Geometry: final body of the model. Coordinates: model frame, mm. A direction names the side the tool comes from. Give positions to 0.01 mm unless a question says otherwise; leave off trailing zeros. Write each loop counter-clockwise with the first axis right and the second up, starting at its lowest first coordinate (ties: lowest second). Pieces come first, ordered by that corner, then holes. Notation, with made-up numbers: M 4.25,62.5 L 52.25,62.5 A21 ccw 52.25,94.5 Z; hole C 22.25,-9 d9. An arc over 180 degrees is marked long. Use a Markdown table: item, result. Add a question column.
(1) Reachability of faces 4 (the cylindrical face through (37.79, -108.4, -99.58)), 5 (the flat face through (60.5, 27, 41)), 6 (the flat face through (11, -2, 150)), 7 (the cylindrical face through (36.1, -77.8, -98.3)), 8 (the cylindrical face through (20.706, -27.169, 86.273)) from +Z, -Z, +X, -X, +Y, -Y: full face, straight path, thin tool, end or side. Return the list, or none.
(2) Pin query (flat end, axial travel): pin 1 Ø3 at (x, y) = (49, -29.5) entering from -Z; pin 2 Ø2 at (x, y) = (24.5, 78) entering from +Z; pin 3 Ø3.5 at (x, z) = (40, 120) entering from +Y. Return the tip coordinate at first contact, or that it passes through.
(3) Cut plane B-B (x = 30). Output: boundary loops of the cut face in (y, z).
(4) Cut plane C-C (z = 32.5). Output: boundary loops of the cut face in (x, y), plus the area to 3 significant figures.
(5) Material intervals for L1, parallel to Z at x = 40, y = -106; L2, parallel to Y at x = 4, z = 0 (3 decimals); L3, parallel to X at y = -108, z = -97, sorted ascending.
(6) Cut plane A-A (y = 0). Output: boundary loops of the cut face in (x, z), plus the area to 3 significant figures.
(7) Cut plane D-D (y = -57.5). Output: boundary loops of the cut face in (x, z).
(8) Draft query along Z for faces 1 (the conical face through (38.568, -75.483, -82.06)), 2 (the conical face through (16.49, 69.66, -82.98)), 3 (the cylindrical face through (37.85, 98.07, -98.34)). Return one class per face: released by +Z, released by -Z, zero draft, split by the parting line, or undercut.
```python
from build123d import *

# Parameters (mm, degrees)
SKETCH1_W                 = 300
SKETCH1_H                 = 260
BOSS_EXTRUDE1_DEPTH       = 60.5
SKETCH2_R                 = 90.45
CUT_EXTRUDE1_DEPTH        = 42
SKETCH9_R                 = 41.51
CUT_EXTRUDE9_DEPTH        = 306
SKETCH12_W                = 39
SKETCH12_H                = 260
CUT_EXTRUDE12_DEPTH       = 14
SKETCH13_W                = 39
SKETCH13_H                = 260
CUT_EXTRUDE13_DEPTH       = 36.45
SKETCH14_W                = 39
SKETCH14_H                = 14
CUT_EXTRUDE14_DEPTH       = 333.506014983
SKETCH15_W                = 22.45
SKETCH15_H                = 260
CUT_EXTRUDE15_DEPTH       = 208.50963833
F_6_0MM_DOWEL_HOLE1_D     = 6
F_6_0MM_DOWEL_HOLE1_DEPTH = 30
F_6_0MM_DOWEL_HOLE1_TIP   = 1.802581857
F_6_0MM_DOWEL_HOLE2_D     = 6
F_6_0MM_DOWEL_HOLE2_DEPTH = 30
F_6_0MM_DOWEL_HOLE2_TIP   = 1.802581857
F_6_0MM_DOWEL_HOLE3_D     = 6
F_6_0MM_DOWEL_HOLE3_DEPTH = 15
F_6_0MM_DOWEL_HOLE3_TIP   = 1.802581857
SKETCH25_W                = 39
SKETCH25_H                = 14
CUT_EXTRUDE16_DEPTH       = 333.506014983
SKETCH26_W                = 257.55
SKETCH26_H                = 240
CUT_EXTRUDE18_DEPTH       = 2.3
F_6_0MM_DOWEL_HOLE4_D     = 6
F_6_0MM_DOWEL_HOLE4_DEPTH = 15
F_6_0MM_DOWEL_HOLE4_TIP   = 1.802581857
SKETCH32_R                = 2.25
CUT_EXTRUDE19_DEPTH       = 57
SKETCH33_R                = 95.95
SKETCH33_R_2              = 91.95
CUT_EXTRUDE21_DEPTH       = 2.3


with BuildPart() as part:
    # Sketch1 → Boss-Extrude1 (new body)
    with BuildSketch(Plane(origin=(0, 0, 0), x_dir=(0, 0, -1), z_dir=(1, 0, 0))):
        Rectangle(SKETCH1_W, SKETCH1_H)
    extrude(amount=BOSS_EXTRUDE1_DEPTH)

    # Sketch2 → Cut-Extrude1 (cut)
    with BuildSketch(Plane(origin=(0, 0, 0), x_dir=(0, 0, -1), z_dir=(1, 0, 0))):
        with Locations(Location((0, 0, 0), (0, 0, 180))):
            Circle(SKETCH2_R)
    extrude(amount=CUT_EXTRUDE1_DEPTH, mode=Mode.SUBTRACT)

    # Sketch9 → Cut-Extrude9 (cut)
    with BuildSketch(Plane(origin=(0, 0, 0), x_dir=(0, 0, -1), z_dir=(1, 0, 0))):
        with Locations(Location((0, 0, 0), (0, 0, 180))):
            Circle(SKETCH9_R)
    extrude(amount=CUT_EXTRUDE9_DEPTH, mode=Mode.SUBTRACT)

    # Sketch12 → Cut-Extrude12 (cut)
    with BuildSketch(Plane.XY.offset(150)):
        with Locations((41, 0)):
            Rectangle(SKETCH12_W, SKETCH12_H)
    extrude(amount=-CUT_EXTRUDE12_DEPTH, mode=Mode.SUBTRACT)

    # Sketch13 → Cut-Extrude13 (cut)
    with BuildSketch(Plane(origin=(0, 0, -150), x_dir=(-1, 0, 0), z_dir=(0, 0, -1))):
        with Locations((-41, 0)):
            Rectangle(SKETCH13_W, SKETCH13_H)
    extrude(amount=-CUT_EXTRUDE13_DEPTH, mode=Mode.SUBTRACT)

    # Sketch14 → Cut-Extrude14 (cut, through all)
    with BuildSketch(Plane.XY.offset(150)):
        with Locations((41, -123)):
            Rectangle(SKETCH14_W, SKETCH14_H)
    extrude(amount=-CUT_EXTRUDE14_DEPTH, mode=Mode.SUBTRACT)

    # Sketch15 → Cut-Extrude15 (cut, through all)
    with BuildSketch(Plane(origin=(0, 0, 0), x_dir=(0, 0, -1), z_dir=(1, 0, 0))):
        with Locations((138.775, 0)):
            Rectangle(SKETCH15_W, SKETCH15_H)
    extrude(amount=CUT_EXTRUDE15_DEPTH, mode=Mode.SUBTRACT)

    # Ø6.0mm Dowel Hole1
    with Locations(Plane.XY.offset(136)):
        with Locations((38.5, 101), (38.5, -76)):
            Hole(F_6_0MM_DOWEL_HOLE1_D / 2, depth=F_6_0MM_DOWEL_HOLE1_DEPTH)
            with Locations((0, 0, -(F_6_0MM_DOWEL_HOLE1_DEPTH + F_6_0MM_DOWEL_HOLE1_TIP / 2))):  # 118° drill point
                Cone(0, F_6_0MM_DOWEL_HOLE1_D / 2, F_6_0MM_DOWEL_HOLE1_TIP, mode=Mode.SUBTRACT)

    # Ø6.0mm Dowel Hole2
    with Locations(Plane(origin=(0, 0, -113.55), x_dir=(-1, 0, 0), z_dir=(0, 0, -1))):
        with Locations((-38.5, 101), (-38.5, -76)):
            Hole(F_6_0MM_DOWEL_HOLE2_D / 2, depth=F_6_0MM_DOWEL_HOLE2_DEPTH)
            with Locations((0, 0, -(F_6_0MM_DOWEL_HOLE2_DEPTH + F_6_0MM_DOWEL_HOLE2_TIP / 2))):  # 118° drill point
                Cone(0, F_6_0MM_DOWEL_HOLE2_D / 2, F_6_0MM_DOWEL_HOLE2_TIP, mode=Mode.SUBTRACT)

    # Ø6.0mm Dowel Hole3
    with Locations(Plane(origin=(0, -116, 0), x_dir=(-1, 0, 0), z_dir=(0, -1, 0))):
        with Locations((-40, -120), (-40, 97.55)):
            Hole(F_6_0MM_DOWEL_HOLE3_D / 2, depth=F_6_0MM_DOWEL_HOLE3_DEPTH)
            with Locations((0, 0, -(F_6_0MM_DOWEL_HOLE3_DEPTH + F_6_0MM_DOWEL_HOLE3_TIP / 2))):  # 118° drill point
                Cone(0, F_6_0MM_DOWEL_HOLE3_D / 2, F_6_0MM_DOWEL_HOLE3_TIP, mode=Mode.SUBTRACT)

    # Sketch25 → Cut-Extrude16 (cut, through all)
    with BuildSketch(Plane(origin=(0, 0, -150), x_dir=(-1, 0, 0), z_dir=(0, 0, -1))):
        with Locations((-41, 123)):
            Rectangle(SKETCH25_W, SKETCH25_H)
    extrude(amount=-CUT_EXTRUDE16_DEPTH, mode=Mode.SUBTRACT)

    # Sketch26 → Cut-Extrude18 (cut)
    with BuildSketch(Plane(origin=(21.5, 0, 0), x_dir=(0, 0, -1), z_dir=(1, 0, 0))):
        with Locations((-11.225, 0)):
            Rectangle(SKETCH26_W, SKETCH26_H)
        with BuildLine():
            Line((-135.5, 116), (113.05, 116))
            ThreePointArc((113.05, 116), (113.403553391, 115.853553391), (113.55, 115.5))
            Line((113.55, 115.5), (113.55, -115.5))
            ThreePointArc((113.55, -115.5), (113.403553391, -115.853553391), (113.05, -116))
            Line((113.05, -116), (-135.5, -116))
            ThreePointArc((-135.5, -116), (-135.853553391, -115.853553391), (-136, -115.5))
            Line((-136, -115.5), (-136, 115.5))
            ThreePointArc((-136, 115.5), (-135.853553391, 115.853553391), (-135.5, 116))
        make_face(mode=Mode.SUBTRACT)
    extrude(amount=-CUT_EXTRUDE18_DEPTH, mode=Mode.SUBTRACT)

    # Ø6.0mm Dowel Hole4
    with Locations(Plane.ZY):
        with Locations((0, 107.825), (82.598742079, 69.308574014), (82.598742079, -69.308574014), (0, -107.825), (-82.598742079, -69.308574014), (-82.598742079, 69.308574014)):
            Hole(F_6_0MM_DOWEL_HOLE4_D / 2, depth=F_6_0MM_DOWEL_HOLE4_DEPTH)
            with Locations((0, 0, -(F_6_0MM_DOWEL_HOLE4_DEPTH + F_6_0MM_DOWEL_HOLE4_TIP / 2))):  # 118° drill point
                Cone(0, F_6_0MM_DOWEL_HOLE4_D / 2, F_6_0MM_DOWEL_HOLE4_TIP, mode=Mode.SUBTRACT)

    # Sketch32 → Cut-Extrude19 (cut)
    with BuildSketch(Plane(origin=(0, -130, 0), x_dir=(-1, 0, 0), z_dir=(0, -1, 0))):
        with Locations(Location((-9, -9.45, 0), (0, 0, 90))):
            Circle(SKETCH32_R)
    extrude(amount=-CUT_EXTRUDE19_DEPTH, mode=Mode.SUBTRACT)

    # Sketch33 → Cut-Extrude21 (cut)
    with BuildSketch(Plane(origin=(0, 0, 0), x_dir=(0, 0, -1), z_dir=(1, 0, 0))):
        Circle(SKETCH33_R)
        Circle(SKETCH33_R_2, mode=Mode.SUBTRACT)
    extrude(amount=CUT_EXTRUDE21_DEPTH, mode=Mode.SUBTRACT)


solid = part.part
```
Answer list:
| question | item | result |
|---|---|---|
| 1 | face 4 | -Y |
| 1 | face 5 | +Z, -Z, +X, +Y, -Y |
| 1 | face 6 | +Z, +X, -X, +Y, -Y |
| 1 | face 7 | -Z |
| 1 | face 8 | -X |
| 2 | pin 1 | z = -113.55 |
| 2 | pin 2 | z = 136 |
| 2 | pin 3 | y = 116 |
| 3 | outline | M -116,-113.55 L 116,-113.55 L 116,136 L -116,136 Z; hole C 0,0 d180.9 |
| 4 | outline | M 0,-130 L 21.5,-130 L 21.5,-120 L 19.2,-120 L 19.2,-116 L 60.5,-116 L 60.5,-25.82 L 42,-25.82 L 42,-84.41 L 0,-84.41 L 0,-86.01 L 2.3,-86.01 L 2.3,-90.28 L 0,-90.28 Z; M 0,84.41 L 42,84.41 L 42,25.82 L 60.5,25.82 L 60.5,116 L 19.2,116 L 19.2,120 L 21.5,120 L 21.5,130 L 0,130 L 0,90.28 L 2.3,90.28 L 2.3,86.01 L 0,86.01 Z |
| 4 | area | 6,550 mm² |
| 5 | L1 | -113.55 to -100.55, -94.55 to 117, 123 to 136 |
| 5 | L2 | -130 to -110.825, -104.825 to -90.45, 90.45 to 104.825, 110.825 to 130 |
| 5 | L3 | 0 to 37.05, 42.95 to 60.5 |
| 6 | outline | M 0,-127.55 L 21.5,-127.55 L 21.5,-117.55 L 19.2,-117.55 L 19.2,-113.55 L 60.5,-113.55 L 60.5,-41.51 L 42,-41.51 L 42,-90.45 L 0,-90.45 L 0,-91.95 L 2.3,-91.95 L 2.3,-95.95 L 0,-95.95 Z; M 0,90.45 L 42,90.45 L 42,41.51 L 60.5,41.51 L 60.5,136 L 19.2,136 L 19.2,140 L 21.5,140 L 21.5,150 L 0,150 L 0,95.95 L 2.3,95.95 L 2.3,91.95 L 0,91.95 Z |
| 6 | area | 6,530 mm² |
| 7 | outline | M 0,-127.55 L 21.5,-127.55 L 21.5,-117.55 L 19.2,-117.55 L 19.2,-113.55 L 60.5,-113.55 L 60.5,136 L 19.2,136 L 19.2,140 L 21.5,140 L 21.5,150 L 0,150 L 0,76.81 L 2.3,76.81 L 2.3,71.75 L 0,71.75 L 0,69.82 L 42,69.82 L 42,-69.82 L 0,-69.82 L 0,-71.75 L 2.3,-71.75 L 2.3,-76.81 L 0,-76.81 Z |
| 8 | face 1 | released by -Z |
| 8 | face 2 | undercut |
| 8 | face 3 | zero draft |
